from build123d import *

# Parameters (mm, degrees)
F0_W     = 13.4628936648
F0_H     = 16.1730796099
F0_W_2   = 5.4922168999
F0_H_2   = 8.2855048865
F0_W_3   = 5.2812833667
F0_H_3   = 6.5011191182
F0_H_4   = 9.2424242757
F1_DEPTH = 25.4


with BuildPart() as f1:
    # F0 (on Front) → F1 (new body)
    with BuildSketch(Plane.XZ):
        Polygon((-29.0956337333, -67.6122568771), (-29.0956337333, -16.8122568771), (-54.4956337333, -16.8122568771), (-54.4956337333, -23.1622568771), (-54.4956337333, -67.6122568771), align=None)
        with Locations((-42.03697294, -42.1628169715)):
            Rectangle(F0_W, F0_H, mode=Mode.SUBTRACT)
        Polygon((-29.0956337333, 21.2877431229), (-54.4956337333, 21.2877431229), (-54.4956337333, 13.0022382364), (-54.4956337333, 6.5011191182), (-54.4956337333, 0), (-54.4956337333, -5.4398714565), (-54.4956337333, -14.6822957322), (-54.4956337333, -16.8122568771), (-29.0956337333, -16.8122568771), align=None)
        with Locations((-57.2417421832, 17.1449906796)):
            Rectangle(F0_W_2, F0_H_2)
        with Locations((-57.1362754166, 3.2505595591)):
            Rectangle(F0_W_3, F0_H_3)
        with Locations((-57.1362754166, -10.0610835943)):
            Rectangle(F0_W_3, F0_H_4)
    extrude(amount=F1_DEPTH)


solid = f1.part
Input: part model. Units: mm. Frame: model coordinates. A direction names the side the tool comes from. Coordinates: 2 decimals unless noted, no trailing zeros. Loops run counter-clockwise (first coordinate to the right, second up) from the corner with the lowest first, then second, coordinate; pieces in that order, holes last. Notation, with made-up numbers: (4.5, 23) -> (54.5, 23) arc R21 ccw to (54.5, 35) -> close; hole circle Ø5 at (39.5, -39.5). An arc over 180 degrees is marked (long way). Write each question's results on one line, items separated by ' | '. Start each with the question number.
Q1. Section C-C, the plane x = -57. Return the cut outline in (y, z).
Q2. Section B-B, the plane z = -39.5. Return the cut outline in (x, y), plus the area to 3 significant figures.
Q3. Reachability of faces 4 (the flat face through (-59.777, -13, -10)), 5 (the flat face through (-57, -13, 13.002)), 6 (the flat face through (-41, 0, -23)), 7 (the flat face through (-42, -13, -34.076)), 8 (the flat face through (-44, -13, 21.288)) from +Z, -Z, +X, -X, +Y, -Y: full face, straight path, thin tool, end or side. Return the list, or none.
Q4. Pin query (flat end, axial travel): pin 1 (6 mm diameter, centred on y = -9.5, z = -1.5, fed in from -X); pin 2 (4 mm diameter, centred on y = -20.5, z = -33, fed in from -X); pin 3 (1.6 mm diameter, centred on x = -58, y = -8, fed in from -Z); pin 4 (2 mm diameter, centred on x = -55, z = -16, fed in from -Y). Return the tip coordinate at first contact, or that it passes through.
Q5. Pull-direction query (X, two-part tool) for faces 1 (the flat face through (-29.096, -13, -24)), 2 (the flat face through (-41, -25.4, -23)), 3 (the flat face through (-35.306, -13, -42)); classes: released by +X, released by -X, zero draft, split by the parting line, or undercut.
Q6. Section D-D, the plane y = -17.5. Return the cut outline in (x, z).
Q7. Section A-A, the plane x = -37. Return the cut outline in (y, z), plus the area to 3 significant figures.
Q8. Ray query, line 1 (Z direction, x = -43, y = -20.5); line 2 (X direction, y = -1, z = -41); line 3 (X direction, y = -14, z = 10.5). Return the intervals inside material, ascending. Write a range as from..to.
Found:
1) outline: (-25.4, -14.68) -> (0, -14.68) -> (0, -5.44) -> (-25.4, -5.44) -> close; (-25.4, 0) -> (0, 0) -> (0, 6.5) -> (-25.4, 6.5) -> close; (-25.4, 13) -> (0, 13) -> (0, 21.29) -> (-25.4, 21.29) -> close
2) outline: (-54.5, -25.4) -> (-48.77, -25.4) -> (-48.77, 0) -> (-54.5, 0) -> close; (-35.31, -25.4) -> (-29.1, -25.4) -> (-29.1, 0) -> (-35.31, 0) -> close | area: 303 mm2
3) face 4: -Z, -X, +Y, -Y | face 5: -X, +Y, -Y | face 6: +Z, -Z, +X, -X, +Y | face 7: +Y, -Y | face 8: +Z, +X, -X, +Y, -Y
4) pin 1: x = -59.78 | pin 2: x = -54.5 | pin 3: z = -14.68 | pin 4: y = -25.4
5) face 1: released by +X | face 2: zero draft | face 3: undercut
6) outline: (-59.99, 13) -> (-54.5, 13) -> (-54.5, 6.5) -> (-59.78, 6.5) -> (-59.78, 0) -> (-54.5, 0) -> (-54.5, -5.44) -> (-59.78, -5.44) -> (-59.78, -14.68) -> (-54.5, -14.68) -> (-54.5, -67.61) -> (-29.1, -67.61) -> (-29.1, 21.29) -> (-59.99, 21.29) -> close; hole (-48.77, -50.25) -> (-35.31, -50.25) -> (-35.31, -34.08) -> (-48.77, -34.08) -> close
7) outline: (-25.4, -67.61) -> (0, -67.61) -> (0, -50.25) -> (-25.4, -50.25) -> close; (-25.4, -34.08) -> (0, -34.08) -> (0, 21.29) -> (-25.4, 21.29) -> close | area: 1,850 mm2
8) line 1: -67.61..-50.25, -34.08..21.29 | line 2: -54.5..-48.77, -35.31..-29.1 | line 3: -54.5..-29.1
